Work out the finished part from the listing and answer in its coordinate system (mm). Coordinates: 2 decimals unless noted, no trailing zeros. Write each loop counter-clockwise with the first axis right and the second up, starting at its lowest first coordinate (ties: lowest second). Pieces come first, ordered by that corner, then holes. Notation, with made-up numbers: M 65,73 L 80,73 A19 cw 80,105 Z; hole C 86,15.5 d5. An arc over 180 degrees is marked long. Answer as CSV lines item,"result". Start each with the question number.
(1) A flat-ended cylindrical pin translates along its axis: P1, Ø5.5, axis at x = 139.7, y = 12.7, coming from the -Z side. Find the tip coordinate at first contact, or state that the pin passes through.
(2) A cutting plane is placed at C-C on z = 9. Count the separate pieces of the cut face and the enclosed holes in it, then the cut area to 3 significant figures.
(3) A cutting plane is placed at A-A on x = 139.7. Give the vertices of the cut face in (y, z) (3 decimals), then the cut area to 3 significant figures.
(4) A cutting plane is placed at B-B on y = 50.8. Give the vertices of the cut face in (x, z) (3 decimals).
(5) The mould has two halves that part along Y. Classify faces 1 (the flat face through (103, 101.6, 13)), 2 (the flat face through (100, 52, 0)), 3 (the cylindrical face through (136.53, 12.84, 12.88)): released by +Y, released by -Y, zero draft, split by the parting line, or undercut.
(6) Find the intervals of material crossed by L1, parallel to Y at x = 139.7, z = 15.5 (3 decimals); L2, parallel to Y at x = 78.5, z = 19.75; L3, parallel to X at y = 52.5, z = 9, in increasing order. Write a range as [from, to].
Autodesk Inventor part; units mm, degrees
ref_plane "YZ Plane" through (0, 0, 0) normal (1, 0, 0) x (0, 1, 0)
ref_plane "XZ Plane" through (0, 0, 0) normal (0, 1, 0) x (-1, 0, 0)
ref_plane "XY Plane" through (0, 0, 0) normal (0, 0, 1) x (1, 0, 0)
sketch "Sketch1" plane through (0, 0, 0) normal (0, 0, 1) x (1, 0, 0)
  line L0 (0, 0) -> (203.2, 0)
  line L1 (203.2, 0) -> (203.2, 101.6)
  line L2 (203.2, 101.6) -> (0, 101.6)
  line L3 (0, 101.6) -> (0, 0)
  dimension "d0" = 203.2
  dimension "d1" = 101.6
extrude "Extrusion1" add sketch "Sketch1" along normal blind 25.4
sketch "Sketch2" plane through (0, 0, 25.4) normal (0, 0, 1) x (1, 0, 0)
  line L0 (203.2, 101.6) -> (0, 101.6)
  line L1 (0, 101.6) -> (0, 0)
  circle A0 centre (12.7, 88.9) radius 3.175
  dimension "d4" = 6.35
  dimension "d5" = 12.7
  dimension "d6" = 12.7
extrude "Extrusion2" cut sketch "Sketch2" against normal through all
pattern_linear "Rectangular Pattern1" count 5 spacing 31.75 along (1, 0, 0) count 3 spacing 38.1 along (0, -1, 0) of "Extrusion2"
properties part number "Rectangular Pattern Parameters"
Here are the results:
1,P1,"passes through"
2,separate pieces,"1"
2,enclosed holes,"15"
2,area,"20,200 mm^2"
3,outline,"M 0,0 L 9.525,0 L 9.525,25.4 L 0,25.4 Z; M 15.875,0 L 47.625,0 L 47.625,25.4 L 15.875,25.4 Z; M 53.975,0 L 85.725,0 L 85.725,25.4 L 53.975,25.4 Z; M 92.075,0 L 101.6,0 L 101.6,25.4 L 92.075,25.4 Z"
3,area,"2,100 mm^2"
4,outline,"M 0,0 L 9.525,0 L 9.525,25.4 L 0,25.4 Z; M 15.875,0 L 41.275,0 L 41.275,25.4 L 15.875,25.4 Z; M 47.625,0 L 73.025,0 L 73.025,25.4 L 47.625,25.4 Z; M 79.375,0 L 104.775,0 L 104.775,25.4 L 79.375,25.4 Z; M 111.125,0 L 136.525,0 L 136.525,25.4 L 111.125,25.4 Z; M 142.875,0 L 203.2,0 L 203.2,25.4 L 142.875,25.4 Z"
5,face 1,"released by +Y"
5,face 2,"zero draft"
5,face 3,"undercut"
6,L1,"y = [0, 9.525], [15.875, 47.625], [53.975, 85.725], [92.075, 101.6]"
6,L2,"y = [0, 10.51], [14.89, 48.61], [52.99, 86.71], [91.09, 101.6]"
6,L3,"x = [0, 10.02], [15.38, 41.77], [47.13, 73.52], [78.88, 105.27], [110.63, 137.02], [142.38, 203.2]"
